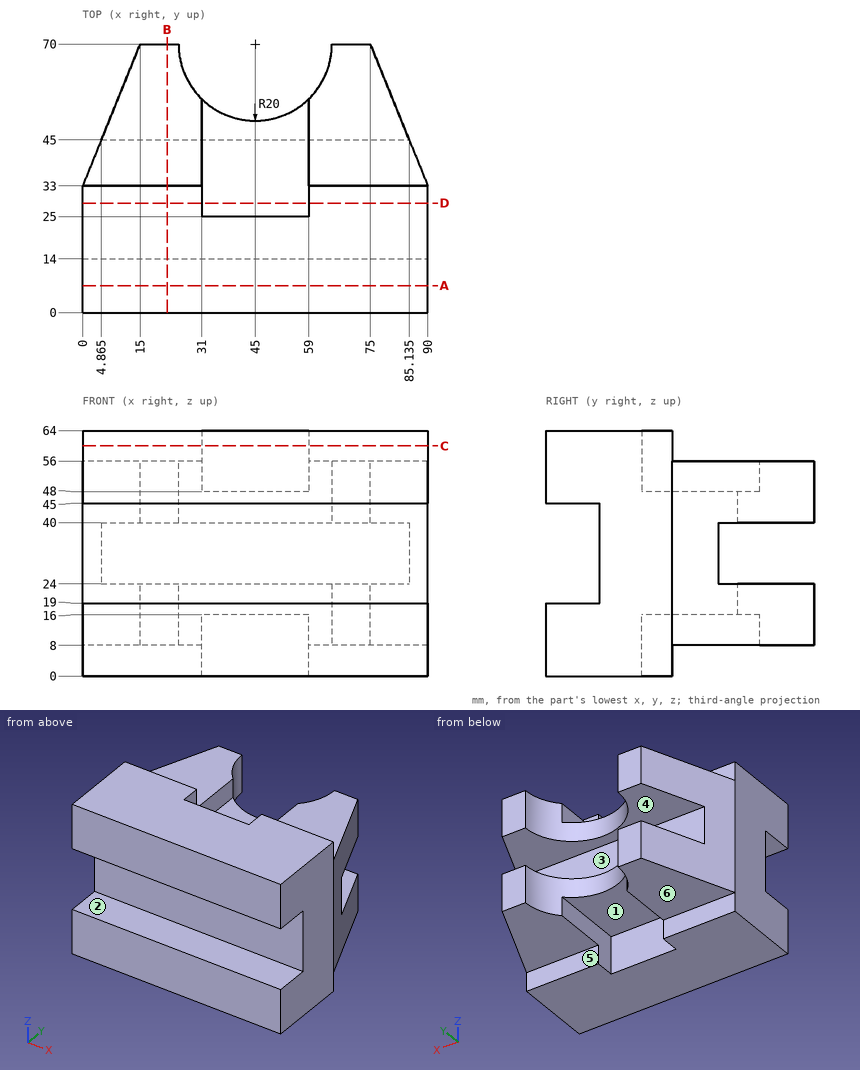
Job drawing, mm, ordinate dimensions from the low corner. One solid piece. A direction names the side the tool comes from. Coordinates: 2 decimals unless noted, no trailing zeros. Write each loop counter-clockwise with the first axis right and the second up, starting at its lowest first coordinate (ties: lowest second). Pieces come first, ordered by that corner, then holes. Notation, with made-up numbers: M 86,-32 L 142,-32 A31 ccw 142,2 Z; hole C 16.5,8.5 d2. An arc over 180 degrees is marked long. Answer as a JSON object with one key per item and string values. Group by question number.
1) Saw through at A-A (y = 7). Write the cut outline in (x, z).
2) Saw through at B-B (x = 22). Write the cut outline in (y, z).
3) Pin check, flat tips, straight feed: pin 1 Ø1 at (x, z) = (68.5, 37.5) entering from +Y; pin 2 Ø17.5 at (y, z) = (43.5, 53.5) entering from +X; pin 3 Ø1.5 at (y, z) = (62, 10) entering from +X. Stop position of each tip, or through.
4) Saw through at D-D (y = 28.5). Write the cut outline in (x, z), plus the area to 3 significant figures.
5) Mould opens along Z. For the marked faces 4, 5 and 6 say: +Z half, -Z half, draft (parallel to the pull), parting line (faces both ways), or undercut.
6) Wall check: line 1 (Z direction, x = 19, y = 53.5); line 2 (Y direction, x = 32, z = 53); line 3 (Z direction, x = 15.5, y = 8). Give the ranges that are in metal, low to high. Write a range as from..to.
7) Saw through at C-C (z = 60). Write the cut outline in (x, y).
8) Tool access for the marked faces 1, 2 and 3: list every direction of +Z, -Z, +X, -X, +Y, -Y with a clear straight run to the whole face (end or side of a thin tool).
Values follow:
{
 "1": {"outline": "M 0,0 L 90,0 L 90,19 L 0,19 Z; M 0,45 L 90,45 L 90,64 L 0,64 Z"},
 "2": {"outline": "M 0,0 L 33,0 L 33,8 L 70,8 L 70,24 L 45,24 L 45,40 L 70,40 L 70,56 L 33,56 L 33,64 L 0,64 L 0,45 L 14,45 L 14,19 L 0,19 Z"},
 "3": {"pin 1": "stops at y = 45", "pin 2": "stops at x = 89.29", "pin 3": "stops at x = 78.55"},
 "4": {"outline": "M 0,0 L 31,0 L 31,16 L 59,16 L 59,0 L 90,0 L 90,64 L 59,64 L 59,48 L 31,48 L 31,64 L 0,64 Z", "area": "4,860 mm2"},
 "5": {"face 4": "undercut", "face 5": "draft", "face 6": "-Z half"},
 "6": {"line 1": "z = 8..24, 40..56", "line 2": "y = 0..25", "line 3": "z = 0..19, 45..64"},
 "7": {"outline": "M 0,0 L 90,0 L 90,33 L 59,33 L 59,25 L 31,25 L 31,33 L 0,33 Z"},
 "8": {"face 1": "-Z, +Y", "face 2": "+X, -X, -Y", "face 3": "+X, -X, +Y"}
}
